Part print with two shaded views. Sizes in mm from the minimum x, y, z corner. Round coordinates to 2 decimals unless told otherwise and drop trailing zeros. Order: outer loops, then holes, each group sorted by start corner. A loop starts at its lowest first (then second) coordinate and runs counter-clockwise, first axis right, second up. Notation, with made-up numbers: M 67.5,38 L 73.5,38 A27 cw 73.5,58 Z; hole C 54.5,80 d5. An arc over 180 degrees is marked long. One line per question, with ' | ' between items.
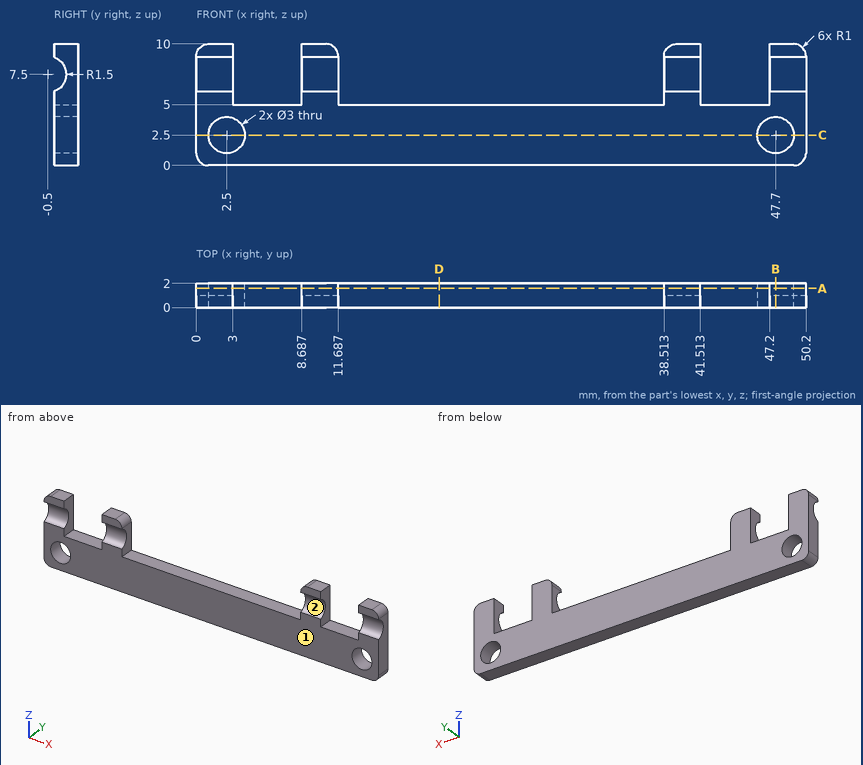
1) Probe line 1 (X direction, y = 0.95, z = 6); line 2 (X direction, y = 0.55, z = 2.5); line 3 (Z direction, x = 2.5, y = 1.35). List the from-to ranges inside material, lowest first. Write a range as [from, to].
The answers:
line 1: x = [0, 3], [8.69, 11.69], [38.51, 41.51], [47.2, 50.2] | line 2: x = [0, 1], [4, 46.2], [49.2, 50.2] | line 3: z = [0, 1], [4, 10]
2) Saw through at B-B (x = 47.7). List the corners of the cut face in (y, z).
The answers:
outline: M 0,0 L 2,0 L 2,1 L 0,1 Z; M 0,4 L 2,4 L 2,10 L 0,10 L 0,8.91 A1.5 cw 0,6.09 Z
3) Drop flat-ended pins along their axis: pin 1 (0.6 mm diameter, centred on x = 25.5, y = 1, fed in from +Z); pin 2 (5 mm diameter, centred on x = 34, z = 8, fed in from +Y). Give the stop position or say it passes through.
The answers:
pin 1: stops at z = 5 | pin 2: passes through
4) Saw through at C-C (z = 2.5). List the corners of the cut face in (x, y).
The answers:
outline: M 0,0 L 1,0 L 1,2 L 0,2 Z; M 4,0 L 46.2,0 L 46.2,2 L 4,2 Z; M 49.2,0 L 50.2,0 L 50.2,2 L 49.2,2 Z
5) Two-plate mould, pull along Z, no slides. Class the marked faces 1 and 2: released by +Z, released by -Z, zero draft, split by the parting line, or undercut.
The answers:
face 1: zero draft | face 2: undercut
6) Saw through at A-A (y = 1.6). List the corners of the cut face in (x, z).
The answers:
outline: M 0,1 A1 ccw 1,0 L 49.2,0 A1 ccw 50.2,1 L 50.2,9 A1 ccw 49.2,10 L 47.2,10 L 47.2,5 L 41.51,5 L 41.51,10 L 39.51,10 A1 ccw 38.51,9 L 38.51,5 L 11.69,5 L 11.69,9 A1 ccw 10.69,10 L 8.69,10 L 8.69,5 L 3,5 L 3,10 L 1,10 A1 ccw 0,9 Z; hole C 2.5,2.5 d3; hole C 47.7,2.5 d3
7) Saw through at D-D (x = 20). List the corners of the cut face in (y, z).
The answers:
outline: M 0,0 L 2,0 L 2,5 L 0,5 Z
